Verification items for the finished model (mm, model axes). Give positions to 0.01 mm unless a question says otherwise; leave off trailing zeros. Loops run counter-clockwise (first coordinate to the right, second up) from the corner with the lowest first, then second, coordinate; pieces in that order, holes last. Notation, with made-up numbers: M 55,-28 L 106,-28 A33 ccw 106,3 Z; hole C 37,13 d8. An arc over 180 degrees is marked long. Use a Markdown table: item, result.
from build123d import *

# Parameters (mm, degrees)
SKETCH1_W           = 4.353701527
SKETCH1_H           = 3.374525205
SKETCH1_H_2         = 3.374525206
SKETCH1_W_2         = 4.353701528
BOSS_EXTRUDE1_DEPTH = 4
SKETCH2_R           = 1.084753974
CUT_EXTRUDE6_DEPTH  = 13.498101


with BuildPart() as part:
    # Sketch1 → Boss-Extrude1 (new body)
    with BuildSketch(Plane(origin=(0, 0, 0), x_dir=(1, 0, 0), z_dir=(0, 1, 0))):
        Polygon((4.353701527, 3.374525206), (4.353701527, 0), (54.259673219, 0), (54.259673219, 3.374525206), (54.259673219, 6.749050412), (54.259673219, 10.123575618), (54.259673219, 13.498100823), (4.353701527, 13.498100823), (4.353701527, 10.123575618), (4.353701527, 6.749050412), align=None)
        with Locations((2.176850764, 11.810838221)):
            Rectangle(SKETCH1_W, SKETCH1_H)
        with Locations((2.176850764, 1.687262603)):
            Rectangle(SKETCH1_W, SKETCH1_H_2)
        with Locations((56.436523983, 11.810838221)):
            Rectangle(SKETCH1_W_2, SKETCH1_H)
        with Locations((56.436523983, 1.687262603)):
            Rectangle(SKETCH1_W_2, SKETCH1_H_2)
    extrude(amount=BOSS_EXTRUDE1_DEPTH)

    # Sketch2 → Cut-Extrude6 (cut)
    with BuildSketch(Plane.XY):
        with Locations((2.176850764, 2)):
            Circle(SKETCH2_R)
        with Locations(Location((56.436523983, 2, 0), (0, 0, 180))):
            Circle(SKETCH2_R)
    extrude(amount=-CUT_EXTRUDE6_DEPTH, mode=Mode.SUBTRACT)


solid = part.part
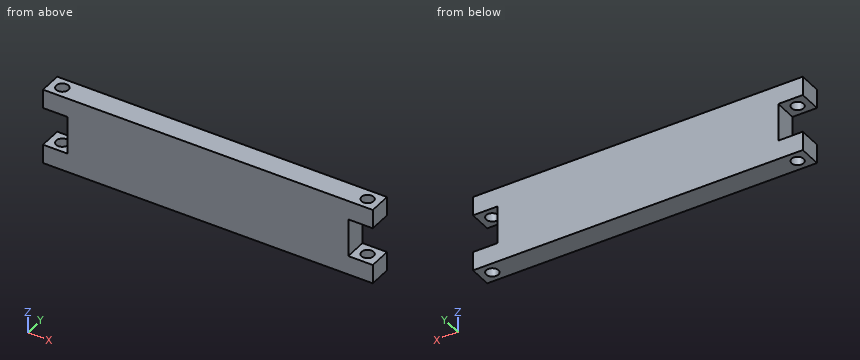
(1) Material ranges on line 1 (X direction, y = 2.2, z = -11.75); line 2 (Z direction, x = 55, y = 0.75); line 3 (X direction, y = 1.85, z = -6), recorded low to high.
Results below:
| item | result |
|---|---|
| line 1 | 0 to 1.11, 3.24 to 55.37, 57.5 to 58.61 |
| line 2 | -13.5 to -10.12, -3.37 to 0 |
| line 3 | 4.35 to 54.26 |
(2) Cross-section at C-C on z = -5.75. Record the cut outline in (x, y), then the cut area to 3 significant figures.
Results below:
| item | result |
|---|---|
| outline | M 4.35,0 L 54.26,0 L 54.26,4 L 4.35,4 Z |
| area | 200 mm^2 |
(3) Cross-section at A-A on y = 2. Record the cut outline in (x, z).
Results below:
| item | result |
|---|---|
| outline | M 0,-13.5 L 1.09,-13.5 L 1.09,-10.12 L 0,-10.12 Z; M 0,-3.37 L 1.09,-3.37 L 1.09,0 L 0,0 Z; M 3.26,-13.5 L 55.35,-13.5 L 55.35,-10.12 L 54.26,-10.12 L 54.26,-3.37 L 55.35,-3.37 L 55.35,0 L 3.26,0 L 3.26,-3.37 L 4.35,-3.37 L 4.35,-10.12 L 3.26,-10.12 Z; M 57.52,-13.5 L 58.61,-13.5 L 58.61,-10.12 L 57.52,-10.12 Z; M 57.52,-3.37 L 58.61,-3.37 L 58.61,0 L 57.52,0 Z |
(4) Cross-section at B-B on z = -1.25. Record the cut outline in (x, y).
Results below:
| item | result |
|---|---|
| outline | M 0,0 L 58.61,0 L 58.61,4 L 0,4 Z; hole C 2.18,2 d2.17; hole C 56.44,2 d2.17 |
(5) Gauge pin test, flat end, axial feed: P1, Ø1.2, axis at y = 1, z = -5, coming from the +X side. Record the tip position at first contact, or that the pin passes through.
Results below:
| item | result |
|---|---|
| P1 | x = 54.26 |
